Part model, mm, in its own coordinate system. A direction names the side the tool comes from. Round coordinates to 2 decimals unless told otherwise and drop trailing zeros. Write each loop counter-clockwise with the first axis right and the second up, starting at its lowest first coordinate (ties: lowest second). Pieces come first, ordered by that corner, then holes. Notation, with made-up numbers: M -38.5,71.5 L -23.5,71.5 A7 cw -23.5,76.5 Z; hole C 42,-38 d1. An arc over 180 degrees is marked long. Answer as a JSON object with one key per item and string values. Group by question number.
1. Drill centre lines: line 1 (Y direction, x = -7, z = -17); line 2 (Y direction, x = 4.75, z = -3.5); line 3 (Z direction, x = 5.5, y = 26). Where is each one in solid material? Low to high. Write a range as from..to.
2. Drop flat-ended pins along their axis: pin 1 (3 mm diameter, centred on x = 7, z = -10, fed in from +Y); pin 2 (9 mm diameter, centred on x = -3, z = -8.5, fed in from +Y); pin 3 (6 mm diameter, centred on x = 4.5, y = 9, fed in from +Z). Give the stop position or say it passes through.
3. Band-saw the part on A-A, the plane z = -8.75. Write the cut outline in (x, y), plus the area to 3 significant figures.
4. Band-saw the part on C-C, the plane y = 31.5. Write the cut outline in (x, z), plus the area to 3 significant figures.
5. Band-saw the part on B-B, the plane x = -11.5. Write the cut outline in (y, z), plus the area to 3 significant figures.
6. Which spindle directions (+Z, -Z, +X, -X, +Y, -Y) get a long thin tool onto all of the face, cutting with end or side? Do faces 1 (the face through (-7.428, 1.789, -14.656)), 2 (the face through (-2, 2.54, 2)), 3 (the face through (2.27, 33.2, -19.7)). Say none if no direction does.
7. Band-saw the part on D-D, the plane x = -1.5. Write the cut outline in (y, z).
8. Two-plate mould, pull along Z, no slides. Class faces 4 (the face through (-4, 1.016, -8)), 5 (the face through (-2, 20, -19.32)), 6 (the face through (3.277, 14.915, -19.696)), 7 (the face through (-2, 19, -20.082)): +Z half, -Z half, draft (parallel to the pull), parting line (faces both ways), or undercut.
from build123d import *

# Parameters (mm, degrees)
SKETCH1_W           = 22.098
SKETCH1_H           = 26.924
BOSS_EXTRUDE1_DEPTH = 2.54
SKETCH2_W           = 22.098
SKETCH2_H           = 0.762
BOSS_EXTRUDE2_DEPTH = 36.068
SKETCH4_R           = 1.651
CUT_EXTRUDE1_DEPTH  = 0.762
SKETCH3_R           = 9.017
CUT_EXTRUDE2_DEPTH  = 1.524
SKETCH5_R           = 1.599485458
CUT_EXTRUDE3_DEPTH  = 1.27
SKETCH6_R           = 1.651
CUT_EXTRUDE4_DEPTH  = 0.762


with BuildPart() as part:
    # Sketch1 → Boss-Extrude1 (new body)
    with BuildSketch(Plane(origin=(0, 0, 0), x_dir=(1, 0, 0), z_dir=(0, 1, 0))):
        with Locations((-1.642418919, 6.620304054)):
            Rectangle(SKETCH1_W, SKETCH1_H)
    extrude(amount=BOSS_EXTRUDE1_DEPTH)

    # Sketch2 → Boss-Extrude2 (add)
    with BuildSketch(Plane(origin=(0, 2.54, 0), x_dir=(1, 0, 0), z_dir=(0, 1, 0))):
        with Locations((-1.642418919, 19.701304054)):
            Rectangle(SKETCH2_W, SKETCH2_H)
    extrude(amount=BOSS_EXTRUDE2_DEPTH)

    # Sketch4 → Cut-Extrude1 (cut)
    with BuildSketch(Plane.XY.offset(-19.320304054)):
        with Locations((-8.168147535, 32.039555002)):
            Circle(SKETCH4_R)
    extrude(amount=-CUT_EXTRUDE1_DEPTH, mode=Mode.SUBTRACT)

    # Sketch3 → Cut-Extrude2 (cut)
    with BuildSketch(Plane(origin=(0, 2.54, 0), x_dir=(1, 0, 0), z_dir=(0, 1, 0))):
        with Locations(Location((-1.941286503, 7.500303052, 0), (0, 0, 270))):
            Circle(SKETCH3_R)
    extrude(amount=-CUT_EXTRUDE2_DEPTH, mode=Mode.SUBTRACT)

    # Sketch5 → Cut-Extrude3 (cut)
    with BuildSketch(Plane(origin=(0, 1.016, 0), x_dir=(1, 0, 0), z_dir=(0, 1, 0))):
        with Locations(Location((-2.007701522, 7.666340599, 0), (0, 0, 270))):
            Circle(SKETCH5_R)
    extrude(amount=-CUT_EXTRUDE3_DEPTH, mode=Mode.SUBTRACT)

    # Sketch6 → Cut-Extrude4 (cut)
    with BuildSketch(Plane.XY.offset(-19.320304054)):
        with Locations((3.491794036, 32.087538301)):
            Circle(SKETCH6_R)
        with Locations((-8.408064028, 13.661951621)):
            Circle(SKETCH6_R)
        with Locations((3.491794036, 13.278085232)):
            Circle(SKETCH6_R)
    extrude(amount=-CUT_EXTRUDE4_DEPTH, mode=Mode.SUBTRACT)


solid = part.part
Worked answers:
{
 "1": {"line 1": "y = 0..2.54", "line 2": "y = 0..1.02", "line 3": "z = -20.08..-19.32"},
 "2": {"pin 1": "stops at y = 2.54", "pin 2": "stops at y = 1.02", "pin 3": "stops at z = -19.32"},
 "3": {"outline": "M -12.69,0 L -3.18,0 L -3.18,1.02 L -10.87,1.02 L -10.87,2.54 L -12.69,2.54 Z; M -0.83,0 L 9.41,0 L 9.41,2.54 L 6.99,2.54 L 6.99,1.02 L -0.83,1.02 Z", "area": "26.5 mm^2"},
 "4": {"outline": "M -12.69,-20.08 L -9.73,-20.08 L -9.73,-19.32 L -12.69,-19.32 Z; M -6.61,-20.08 L 1.95,-20.08 L 1.95,-19.32 L -6.61,-19.32 Z; M 5.03,-20.08 L 9.41,-20.08 L 9.41,-19.32 L 5.03,-19.32 Z", "area": "12.1 mm^2"},
 "5": {"outline": "M 0,-20.08 L 38.61,-20.08 L 38.61,-19.32 L 2.54,-19.32 L 2.54,6.84 L 0,6.84 Z", "area": "95.9 mm^2"},
 "6": {"face 1": "+Y", "face 2": "+Z, +X, -X, +Y", "face 3": "+Z, -Z"},
 "7": {"outline": "M 0,-20.08 L 38.61,-20.08 L 38.61,-19.32 L 2.54,-19.32 L 2.54,-16.51 L 1.02,-16.51 L 1.02,-9.18 L 0,-9.18 Z; M 0,-6.15 L 1.02,-6.15 L 1.02,1.51 L 2.54,1.51 L 2.54,6.84 L 0,6.84 Z"},
 "8": {"face 4": "undercut", "face 5": "+Z half", "face 6": "draft", "face 7": "-Z half"}
}
